Geometry check sheet. Reference: the model listing, model coordinates, mm. Face numbers are marked on the shaded views. A direction names the side the tool comes from. Round coordinates to 2 decimals unless told otherwise and drop trailing zeros. Order: outer loops, then holes, each group sorted by start corner. A loop starts at its lowest first (then second) coordinate and runs counter-clockwise, first axis right, second up.
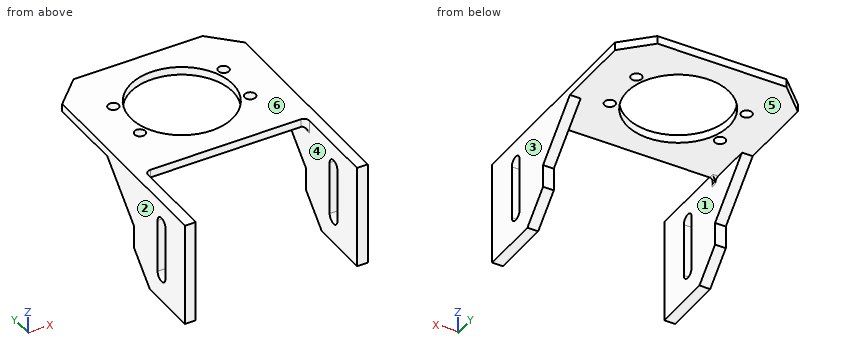
```python
from build123d import *

# Parameters (mm, degrees)
SKETCH_1_R             = 2
SKETCH_1_R_2           = 19
EXTRUDE_1_DEPTH        = 3
EXTRUDE_2_DEPTH        = 4
FILLET_3_R             = 2
FILLET_4_R             = 2
FILLET_3_OF_MIRROR_1_R = 2
FILLET_4_OF_MIRROR_1_R = 2
RIB_1_REACH            = 99.776
SKETCH_4_WALL_W        = 221.83912235
SKETCH_4_WALL_H        = 4


with BuildPart() as part:
    # 草图1 → 凸台-拉伸1 (new body)
    with BuildSketch(Plane.XY):
        Polygon((-24, 28), (24, 28), (34, 18), (34, -28), (-34, -28), (-34, 18), align=None)
        with Locations((20.5, -8.5)):
            Circle(SKETCH_1_R, mode=Mode.SUBTRACT)
        with Locations((20.5, 8.5)):
            Circle(SKETCH_1_R, mode=Mode.SUBTRACT)
        with Locations((-20.5, -8.5)):
            Circle(SKETCH_1_R, mode=Mode.SUBTRACT)
        with Locations((-20.5, 8.5)):
            Circle(SKETCH_1_R, mode=Mode.SUBTRACT)
        Circle(SKETCH_1_R_2, mode=Mode.SUBTRACT)
    extrude(amount=EXTRUDE_1_DEPTH)

    # 草图3 → 凸台-拉伸2 (add)
    with BuildSketch(Plane(origin=(34, 0, 0), x_dir=(0, 0, -1), z_dir=(1, 0, 0))):
        Polygon((-3, -28), (-3, -60.5), (35.720694049, -60.5), (35.720694049, -38), (25.720694049, -28), align=None)
        with BuildLine():
            Line((5.647014868, -43), (25.647014868, -43))
            ThreePointArc((25.647014868, -43), (28.147014868, -45.5), (25.647014868, -48))
            Line((25.647014868, -48), (5.647014868, -48))
            ThreePointArc((5.647014868, -48), (3.147014868, -45.5), (5.647014868, -43))
        make_face(mode=Mode.SUBTRACT)
    extrude_2 = extrude(amount=-EXTRUDE_2_DEPTH)

    # 圆角3
    fillet_3_edges = [part.edges().sort_by_distance(p)[0] for p in [
        (32, -28, 0),
    ]]
    fillet(fillet_3_edges, radius=FILLET_3_R)

    # 圆角4
    fillet_4_edges = [part.edges().sort_by_distance(p)[0] for p in [
        (30, -28, 1.5),
        (30, -27, 0),
    ]]
    fillet(fillet_4_edges, radius=FILLET_4_R)

    # 镜向1: 凸台-拉伸2 across plane
    add(extrude_2.mirror(Plane(origin=(0, 0, 0), x_dir=(0, 0, 1), z_dir=(1, 0, 0))))

    # 圆角3 of 镜向1
    fillet_3_of_mirror_1_edges = [part.edges().sort_by_distance(p)[0] for p in [
        (-32, -28, 0),
    ]]
    fillet(fillet_3_of_mirror_1_edges, radius=FILLET_3_OF_MIRROR_1_R)

    # 圆角4 of 镜向1
    fillet_4_of_mirror_1_edges = [part.edges().sort_by_distance(p)[0] for p in [
        (-30, -28, 1.5),
        (-30, -27, 0),
    ]]
    fillet(fillet_4_of_mirror_1_edges, radius=FILLET_4_OF_MIRROR_1_R)

    # 草图4 wall → 筋1 (add, up to next)
    with BuildSketch(Plane(origin=(34, -19.413465197, -8.586534803), x_dir=(0, -0.707106781187, -0.707106781187), z_dir=(0, 0.707106781187, -0.707106781187)), mode=Mode.PRIVATE) as rib_1_sk1:
        with Locations((0, 2)):
            Rectangle(SKETCH_4_WALL_W, SKETCH_4_WALL_H)
    rib_1_tool1 = extrude(rib_1_sk1.sketch, amount=-RIB_1_REACH, mode=Mode.PRIVATE) - part.part
    rib_1 = rib_1_tool1.solids().sort_by_distance((34, -19.413465197, -8.586534803))[0]
    add(rib_1)

    # 镜向2: 筋1 across plane
    add(rib_1.mirror(Plane(origin=(0, 0, 0), x_dir=(0, 0, 1), z_dir=(1, 0, 0))))


solid = part.part
```
(1) Depth check by flat-ended pin: P1, Ø3, axis at x = -31, z = -23.5, coming from the +Y side; P2, Ø5, axis at x = 20.5, y = 8.5, coming from the -Z side; P3, Ø3.5, axis at x = 14, z = 2, coming from the -Y side. Enter the tip coordinate at first touch or a pass-through.
Returned:
P1: stops at y = -28
P2: stops at z = 0
P3: stops at y = -28
(2) Sectioned sample at B-B, the plane x = 0. Record the cut outline in (y, z), and give its area (3 significant figures).
Returned:
outline: (-28, 0) - (-19, 0) - (-19, 3) - (-28, 3) - close; (19, 0) - (28, 0) - (28, 3) - (19, 3) - close
area: 54.0 mm2
(3) Draft check along X on the marked faces 1, 2, 3 and 4. Enter one of: released by +X, released by -X, zero draft, split by the parting line, or undercut.
Returned:
face 1: undercut
face 2: released by -X
face 3: released by +X
face 4: undercut
(4) Set-up check for the marked faces 5 and 6: record each of +Z, -Z, +X, -X, +Y, -Y from which the full face is reachable in a straight line by a thin tool's end or side.
Returned:
face 5: -Z, +Y
face 6: +Z, +X, -X, +Y, -Y
(5) Sectioned sample at D-D, the plane y = -14. Record the cut outline in (x, z).
Returned:
outline: (-34, -3.17) - (-30, -3.17) - (-30, 0) - (-12.85, 0) - (-12.85, 3) - (-34, 3) - close; (12.85, 0) - (30, 0) - (30, -3.17) - (34, -3.17) - (34, 3) - (12.85, 3) - close
(6) Sectioned sample at A-A, the plane y = 0. Record the cut outline in (x, z).
Returned:
outline: (-34, 0) - (-19, 0) - (-19, 3) - (-34, 3) - close; (19, 0) - (34, 0) - (34, 3) - (19, 3) - close
(7) Material ranges on line 1 (Y direction, x = 20.5, z = 2.2); line 2 (X direction, y = -48.5, z = -3.5); line 3 (Z direction, x = -15.5, y = 14.5), recorded low to high.
Returned:
line 1: y = -28 to -10.5, -6.5 to 6.5, 10.5 to 28
line 2: x = -34 to -30, 30 to 34
line 3: z = 0 to 3
(8) Sectioned sample at C-C, the plane y = -45.5. Record the cut outline in (x, z).
Returned:
outline: (-34, -35.72) - (-30, -35.72) - (-30, -28.15) - (-34, -28.15) - close; (-34, -3.15) - (-30, -3.15) - (-30, 3) - (-34, 3) - close; (30, -35.72) - (34, -35.72) - (34, -28.15) - (30, -28.15) - close; (30, -3.15) - (34, -3.15) - (34, 3) - (30, 3) - close
